CAD build for the part. Positions are in the model's coordinates, mm. Face numbers are marked on the shaded views. Round coordinates to 2 decimals unless told otherwise and drop trailing zeros. Loops run counter-clockwise (first coordinate to the right, second up) from the corner with the lowest first, then second, coordinate; pieces in that order, holes last.
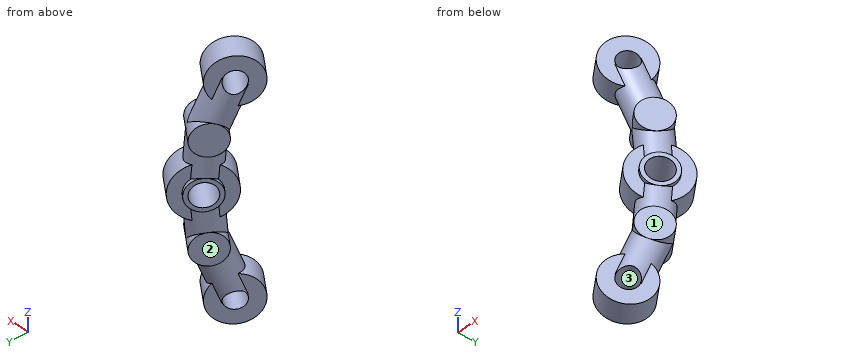
from build123d import *

# Parameters (mm, degrees)
ARCO_1_PROFILE_R           = 4
ARCO_2_PROFILE_R           = 4
ARCO_3_PROFILE_R           = 4
ARCO_4_PROFILE_R           = 4
ARCO_CODO_1_PROFILE_R      = 4
ARCO_CODO_2_PROFILE_R      = 4
ARCO_CODO_3_PROFILE_R      = 4
BOSS_IZQ_PROFILE_R         = 6
BOSS_DCHO_PROFILE_R        = 6
BOSS_CENTRO_PROFILE_R      = 7
PIVOTE_IZQ_PROFILE_R       = 2.5
PIVOTE_DCHO_PROFILE_R      = 2.5
TALADRO_TORNILLO_PROFILE_R = 3


with BuildPart() as part:
    # Arco_1: sweep along a curve in space
    with BuildLine() as arco_1_path:
        Line((-231.363734357, 348.939584198, -26), (-228.368101152, 352.942855573, -13))
    # Arco_1 profile (on start of the path) → Arco_1 (sweep)
    with BuildSketch(Plane(origin=(-231.363734357, 348.939584198, -26), x_dir=(0, 0.9557113836787837, -0.29430554039430606), z_dir=(0.215073929957754, 0.28741813449044995, 0.9333456062030596))):
        Circle(ARCO_1_PROFILE_R)
    sweep(path=arco_1_path.line)

    # Arco_2: sweep along a curve in space
    with BuildLine() as arco_2_path:
        Line((-228.368101152, 352.942855573, -13), (-227.768974511, 353.743509848, 0))
    # Arco_2 profile (on start of the path) → Arco_2 (sweep)
    with BuildSketch(Plane(origin=(-228.368101152, 352.942855573, -13), x_dir=(0, 0.9981087890283697, -0.06147231298984599), z_dir=(0.04595091574946005, 0.06140737971093147, 0.9970544855015816))):
        Circle(ARCO_2_PROFILE_R)
    sweep(path=arco_2_path.line)

    # Arco_3: sweep along a curve in space
    with BuildLine() as arco_3_path:
        Line((-227.768974511, 353.743509848, 0), (-228.368101152, 352.942855573, 13))
    # Arco_3 profile (on start of the path) → Arco_3 (sweep)
    with BuildSketch(Plane(origin=(-227.768974511, 353.743509848, 0), x_dir=(0, 0.9981087890283697, 0.06147231298984599), z_dir=(-0.04595091574946005, -0.06140737971093147, 0.9970544855015816))):
        Circle(ARCO_3_PROFILE_R)
    sweep(path=arco_3_path.line)

    # Arco_4: sweep along a curve in space
    with BuildLine() as arco_4_path:
        Line((-228.368101152, 352.942855573, 13), (-231.363734357, 348.939584198, 26))
    # Arco_4 profile (on start of the path) → Arco_4 (sweep)
    with BuildSketch(Plane(origin=(-228.368101152, 352.942855573, 13), x_dir=(0, 0.9557113836787837, 0.29430554039430606), z_dir=(-0.215073929957754, -0.28741813449044995, 0.9333456062030596))):
        Circle(ARCO_4_PROFILE_R)
    sweep(path=arco_4_path.line)

    # Arco_codo_1: sweep along a curve in space
    with BuildLine() as arco_codo_1_path:
        Line((-225.165484052, 350.546349009, -13), (-231.570718252, 355.339362137, -13))
    # Arco_codo_1 profile (on start of the path) → Arco_codo_1 (sweep)
    with BuildSketch(Plane(origin=(-225.165484052, 350.546349009, -13), x_dir=(-0.5991266409502999, -0.8006542750173826, 0), z_dir=(-0.8006542750173826, 0.5991266409502999, 0))):
        Circle(ARCO_CODO_1_PROFILE_R)
    sweep(path=arco_codo_1_path.line)

    # Arco_codo_2: sweep along a curve in space
    with BuildLine() as arco_codo_2_path:
        Line((-224.566357411, 351.347003284, 0), (-230.971591611, 356.140016412, 0))
    # Arco_codo_2 profile (on start of the path) → Arco_codo_2 (sweep)
    with BuildSketch(Plane(origin=(-224.566357411, 351.347003284, 0), x_dir=(-0.5991266409502999, -0.8006542750173826, 0), z_dir=(-0.8006542750173826, 0.5991266409502999, 0))):
        Circle(ARCO_CODO_2_PROFILE_R)
    sweep(path=arco_codo_2_path.line)

    # Arco_codo_3: sweep along a curve in space
    with BuildLine() as arco_codo_3_path:
        Line((-225.165484052, 350.546349009, 13), (-231.570718252, 355.339362137, 13))
    # Arco_codo_3 profile (on start of the path) → Arco_codo_3 (sweep)
    with BuildSketch(Plane(origin=(-225.165484052, 350.546349009, 13), x_dir=(-0.5991266409502999, -0.8006542750173826, 0), z_dir=(-0.8006542750173826, 0.5991266409502999, 0))):
        Circle(ARCO_CODO_3_PROFILE_R)
    sweep(path=arco_codo_3_path.line)

    # Boss_izq: sweep along a curve in space
    with BuildLine() as boss_izq_path:
        Line((-228.961771531, 347.142204275, -26), (-233.765697182, 350.736964121, -26))
    # Boss_izq profile (on start of the path) → Boss_izq (sweep)
    with BuildSketch(Plane(origin=(-228.961771531, 347.142204275, -26), x_dir=(-0.5991266409502979, -0.8006542750173841, 0), z_dir=(-0.8006542750173841, 0.5991266409502979, 0))):
        Circle(BOSS_IZQ_PROFILE_R)
    sweep(path=boss_izq_path.line)

    # Boss_dcho: sweep along a curve in space
    with BuildLine() as boss_dcho_path:
        Line((-228.961771531, 347.142204275, 26), (-233.765697182, 350.736964121, 26))
    # Boss_dcho profile (on start of the path) → Boss_dcho (sweep)
    with BuildSketch(Plane(origin=(-228.961771531, 347.142204275, 26), x_dir=(-0.5991266409502979, -0.8006542750173841, 0), z_dir=(-0.8006542750173841, 0.5991266409502979, 0))):
        Circle(BOSS_DCHO_PROFILE_R)
    sweep(path=boss_dcho_path.line)

    # Boss_centro: sweep along a curve in space
    with BuildLine() as boss_centro_path:
        Line((-225.367011686, 351.946129925, 0), (-230.170937336, 355.540889771, 0))
    # Boss_centro profile (on start of the path) → Boss_centro (sweep)
    with BuildSketch(Plane(origin=(-225.367011686, 351.946129925, 0), x_dir=(-0.5991266409502979, -0.8006542750173841, 0), z_dir=(-0.8006542750173841, 0.5991266409502979, 0))):
        Circle(BOSS_CENTRO_PROFILE_R)
    sweep(path=boss_centro_path.line)

    # Pivote_izq: sweep along a curve in space
    with BuildLine() as pivote_izq_path:
        Line((-228.161117256, 346.543077634, -26), (-234.566351457, 351.336090762, -26))
    # Pivote_izq profile (on start of the path) → Pivote_izq (sweep, cut)
    with BuildSketch(Plane(origin=(-228.161117256, 346.543077634, -26), x_dir=(-0.5991266409502999, -0.8006542750173826, 0), z_dir=(-0.8006542750173826, 0.5991266409502999, 0))):
        Circle(PIVOTE_IZQ_PROFILE_R)
    sweep(path=pivote_izq_path.line, mode=Mode.SUBTRACT)

    # Pivote_dcho: sweep along a curve in space
    with BuildLine() as pivote_dcho_path:
        Line((-228.161117256, 346.543077634, 26), (-234.566351457, 351.336090762, 26))
    # Pivote_dcho profile (on start of the path) → Pivote_dcho (sweep, cut)
    with BuildSketch(Plane(origin=(-228.161117256, 346.543077634, 26), x_dir=(-0.5991266409502999, -0.8006542750173826, 0), z_dir=(-0.8006542750173826, 0.5991266409502999, 0))):
        Circle(PIVOTE_DCHO_PROFILE_R)
    sweep(path=pivote_dcho_path.line, mode=Mode.SUBTRACT)

    # Taladro_tornillo: sweep along a curve in space
    with BuildLine() as taladro_tornillo_path:
        Line((-224.566357411, 351.347003284, 0), (-230.971591611, 356.140016412, 0))
    # Taladro_tornillo profile (on start of the path) → Taladro_tornillo (sweep, cut)
    with BuildSketch(Plane(origin=(-224.566357411, 351.347003284, 0), x_dir=(-0.5991266409502999, -0.8006542750173826, 0), z_dir=(-0.8006542750173826, 0.5991266409502999, 0))):
        Circle(TALADRO_TORNILLO_PROFILE_R)
    sweep(path=taladro_tornillo_path.line, mode=Mode.SUBTRACT)


solid = part.part
Item 1: Cut at A-A (z = -2). List the corners of the cut face in (x, y).
Verdict:
outline: (-234.19, 350.17) - (-229.39, 346.58) - (-227.44, 349.17) - (-226.64, 348.57) - (-225.91, 349.56) - (-232.31, 354.35) - (-233.05, 353.37) - (-232.25, 352.77) - close; (-229.63, 357.93) - (-223.23, 353.14) - (-222.49, 354.12) - (-223.29, 354.72) - (-221.35, 357.32) - (-226.15, 360.91) - (-228.1, 358.31) - (-228.9, 358.91) - close
Item 2: Wall check: L1, parallel to Z at x = -228, y = 350.75; L2, parallel to Z at x = -235, y = 346.25; L3, parallel to Y at x = -231.25, z = -24.5. Give the ranges that are in metal, low to high.
Verdict:
L1: z = -30.9 to -1.6, 1.6 to 30.9
L2: z = -30.15 to -21.85, 21.85 to 30.15
L3: y = 344.08 to 346.36, 351.35 to 354.1
Item 3: Flat gauge pins, fed straight in: P1, Ø5, axis at y = 353.5, z = 13, coming from the +X side; P2, Ø3, axis at x = -228.5, z = 16, coming from the +Y side; P3, Ø8, axis at x = -230, y = 357.5, coming from the -Z side. Where does each tip first touch, or does it go through?
Verdict:
P1: stops at x = -222.77
P2: stops at y = 358.19
P3: stops at z = -30.64
Item 4: Mould opens along Y. For the marked faces 1, 2 and 3 say: released by +Y, released by -Y, zero draft, split by the parting line, or undercut.
Verdict:
face 1: released by -Y
face 2: released by +Y
face 3: undercut
